The drawing under review shows one solid part. Ordinate dimensions are in mm from its lowest x, y, z. A direction names the side the tool comes from. Give positions to 0.01 mm unless a question says otherwise; leave off trailing zeros. Order: outer loops, then holes, each group sorted by start corner. A loop starts at its lowest first (then second) coordinate and runs counter-clockwise, first axis right, second up. Notation, with made-up numbers: (71, -25) -> (110, -25) arc R32 cw to (110, 5) -> close; hole circle Ø6 at (-17.75, -17.5). An arc over 180 degrees is marked (long way). Return JSON: item names as keys, results as strings. Group by question number.
1) Add section C-C (z = 27.25). Give the boundary of the cut face in (x, y).
2) The part is to be moulded in two halves that separate along X. For the marked faces 4, 5, 6 and 7, say which applies: released by +X, released by -X, zero draft, split by the parting line, or undercut.
3) Add section A-A (x = 14). Give the boundary of the cut face in (y, z).
4) Add section D-D (x = 3). Give the boundary of the cut face in (y, z), then the cut area to 3 significant figures.
5) Add section B-B (z = 7). Give the boundary of the cut face in (x, y) (1 decimal).
6) To check wall thickness, follow line 1 along X through (y, z) = (16.5, 22.75); line 2 along X through (y, z) = (10.75, 4.75); line 3 along Z through (x, y) = (11.5, 15.75). State the ranges of each line that lie inside material, in increasing order.
7) For the marked faces 1, 2 and 3, list the 3-axis set-ups (+Z, -Z, +X, -X, +Y, -Y) from which the entire face can be reached by the end or side of a thin tool; tool diameter is ignored.
8) Insertion check: P1, Ø13.5, axis at x = 28, z = 21, coming from the +Y side; P2, Ø3, axis at x = 5.5, z = 26, coming from the -Y side; P3, Ø4, axis at y = 2, z = 8, coming from the -X side; P4, Ø3, axis at x = 26, z = 15.5, coming from the +Y side. Each pin has a flat end and moves straight along its axis. Give the tip position at first contact, or say it passes through.
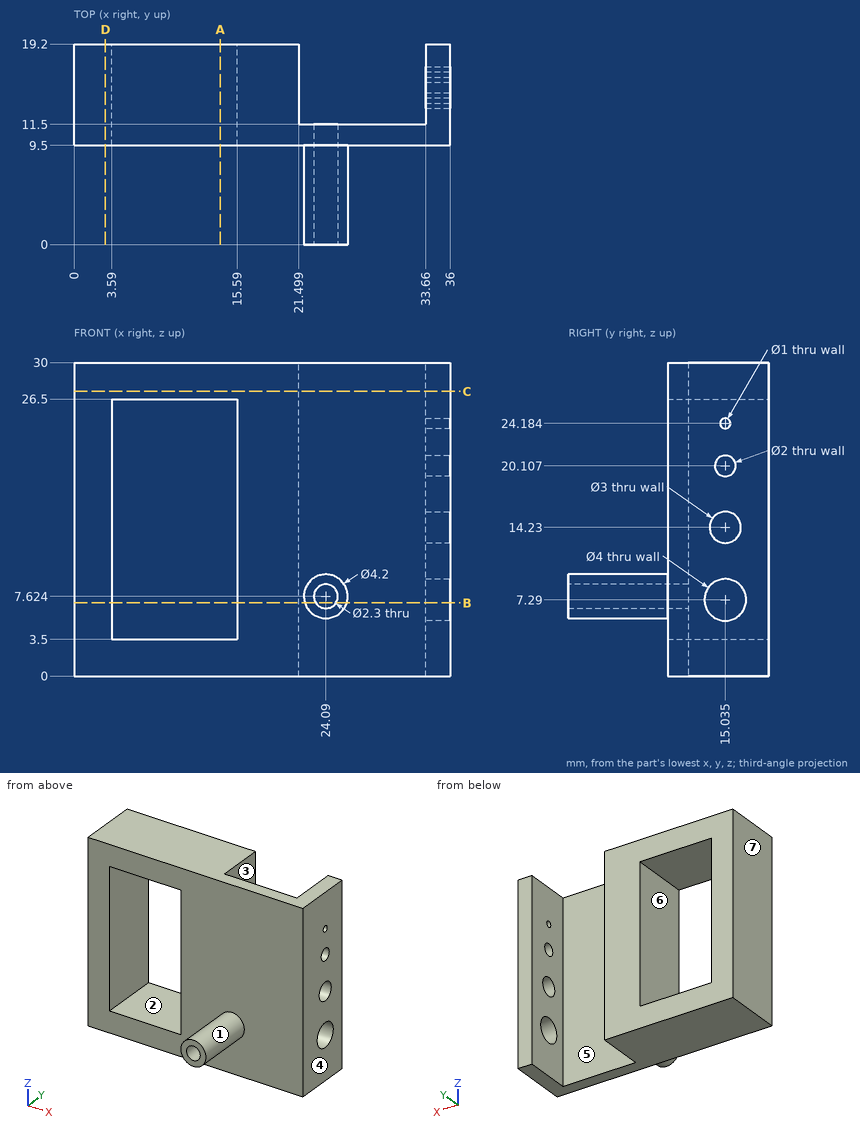
Evaluation:
{
 "1": {"outline": "(0, 9.5) -> (36, 9.5) -> (36, 19.2) -> (33.66, 19.2) -> (33.66, 11.5) -> (21.5, 11.5) -> (21.5, 19.2) -> (0, 19.2) -> close"},
 "2": {"face 4": "released by +X", "face 5": "undercut", "face 6": "undercut", "face 7": "released by -X"},
 "3": {"outline": "(9.5, 0) -> (19.2, 0) -> (19.2, 3.5) -> (9.5, 3.5) -> close; (9.5, 26.5) -> (19.2, 26.5) -> (19.2, 30) -> (9.5, 30) -> close"},
 "4": {"outline": "(9.5, 0) -> (19.2, 0) -> (19.2, 30) -> (9.5, 30) -> close", "area": "291 mm^2"},
 "5": {"outline": "(0, 9.5) -> (3.6, 9.5) -> (3.6, 19.2) -> (0, 19.2) -> close; (15.6, 9.5) -> (22.1, 9.5) -> (22.1, 0) -> (23.1, 0) -> (23.1, 11.5) -> (21.5, 11.5) -> (21.5, 19.2) -> (15.6, 19.2) -> close; (25.1, 0) -> (26.1, 0) -> (26.1, 9.5) -> (36, 9.5) -> (36, 13.1) -> (33.7, 13.1) -> (33.7, 11.5) -> (25.1, 11.5) -> close; (33.7, 17) -> (36, 17) -> (36, 19.2) -> (33.7, 19.2) -> close"},
 "6": {"line 1": "0 to 3.59, 15.59 to 21.5, 33.66 to 36", "line 2": "0 to 3.59, 15.59 to 36", "line 3": "0 to 3.5, 26.5 to 30"},
 "7": {"face 1": "-Y", "face 2": "+Y, -Y", "face 3": "+Z, -Z, +Y"},
 "8": {"P1": "y = 19.2", "P2": "y = 9.5", "P3": "x = 21.99", "P4": "y = 11.5"}
}
